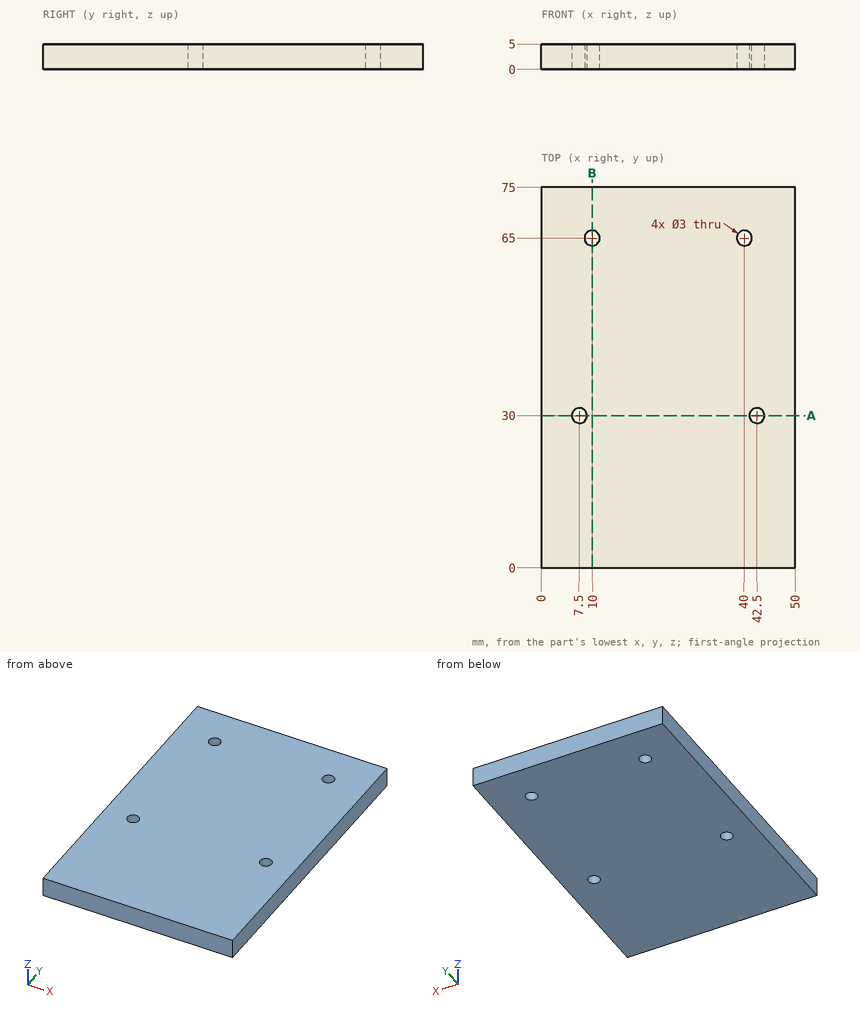
For this review, use the dimensioned drawing (mm, ordinates from the lowest corner) and the shaded views. Give positions to 0.01 mm unless a question says otherwise; leave off trailing zeros. Order: outer loops, then holes, each group sorted by start corner. A loop starts at its lowest first (then second) coordinate and runs counter-clockwise, first axis right, second up. Notation, with made-up numbers: (49.25, 36.25) - (104.25, 36.25) arc R17 cw to (104.25, 63.25) - close; hole circle Ø4 at (-31.5, 65.5). An arc over 180 degrees is marked (long way). Use a Markdown table: item, result. Add a question column.
(1) Add section B-B on x = 10. Give the boundary of the cut face in (y, z).
(2) Wall thickness on probe 1 along X at (y, z) = (65, 3.6); probe 2 along Y at (x, z) = (10, 3.2); probe 3 along Y at (x, z) = (8, 3.1): over which ranges is each line inside the solid? List them lowest first. Write a range as [from, to].
(3) Add section A-A on y = 30. Give the boundary of the cut face in (x, z), then the cut area to 3 significant figures.
(4) Clearance check with a flat-ended pin moving along its axis: P1, Ø4, axis at x = 40, y = 65, coming from the +Z side. State where the tip first meets the part, or that it passes through.
Report:
| question | item | result |
|---|---|---|
| 1 | outline | (0, 0) - (63.5, 0) - (63.5, 5) - (0, 5) - close; (66.5, 0) - (75, 0) - (75, 5) - (66.5, 5) - close |
| 2 | probe 1 | x = [0, 8.5], [11.5, 38.5], [41.5, 50] |
| 2 | probe 2 | y = [0, 63.5], [66.5, 75] |
| 2 | probe 3 | y = [0, 28.59], [31.41, 75] |
| 3 | outline | (0, 0) - (6, 0) - (6, 5) - (0, 5) - close; (9, 0) - (41, 0) - (41, 5) - (9, 5) - close; (44, 0) - (50, 0) - (50, 5) - (44, 5) - close |
| 3 | area | 220 mm² |
| 4 | P1 | stops at z = 5 |
